The listing builds one solid part. Answer for the finished solid, in the listing's coordinates (mm). Coordinates: 2 decimals unless noted, no trailing zeros. Order: outer loops, then holes, each group sorted by start corner. A loop starts at its lowest first (then second) coordinate and runs counter-clockwise, first axis right, second up. Notation, with made-up numbers: (15.25, -28.5) -> (61.25, -28.5) arc R15 cw to (61.25, -11.5) -> close; hole circle Ø9 at (-29.75, 42.25). An arc over 180 degrees is marked (long way). One line per question, with ' | ' between items.
from build123d import *

# Parameters (mm, degrees)
SKETCH1_R           = 2.5
BOSS_EXTRUDE1_DEPTH = 4
CHAMFER1_SIZE       = 0.2


with BuildPart() as part:
    # Sketch1 → Boss-Extrude1 (new body)
    with BuildSketch(Plane(origin=(0, 0, 0), x_dir=(1, 0, 0), z_dir=(0, 1, 0))):
        Polygon((-2.309401077, 4), (-4.618802154, 0), (-2.309401077, -4), (2.309401077, -4), (4.618802154, 0), (2.309401077, 4), align=None)
        with Locations(Location((0, 0, 0), (0, 0, 270))):
            Circle(SKETCH1_R, mode=Mode.SUBTRACT)
    extrude(amount=BOSS_EXTRUDE1_DEPTH)

    # Chamfer1
    chamfer1_edges = [part.edges().sort_by_distance(p)[0] for p in [
        (0, 0, -2.5),
        (0, 4, -2.5),
    ]]
    chamfer(chamfer1_edges, length=CHAMFER1_SIZE)

    # Sketch2 → Cut-Revolve1 (revolve, cut)
    with BuildSketch(Plane.XY):
        Polygon((-4, 4), (-5, 3), (-5, 4), align=None)
        Polygon((-5, 0), (-4, 0), (-5, 1), align=None)
    revolve(axis=Axis((0, 0, 0), (0, 1, 0)), mode=Mode.SUBTRACT)


solid = part.part
Item 1: Section A-A, the plane y = 2.25 is taken. Give the vertices of the cut face in (x, z).
Computed values:
outline: (-4.62, 0) -> (-2.31, -4) -> (2.31, -4) -> (4.62, 0) -> (2.31, 4) -> (-2.31, 4) -> close; hole circle Ø5 at (0, 0)
Item 2: Find the intervals of material crossed by L1, parallel to Z at x = -1, y = 2.75; L2, parallel to X at y = 3, z = -1.75; L3, parallel to Z at x = -1.25, y = 3.1, in increasing order.
Computed values:
L1: z = -4 to -2.29, 2.29 to 4 | L2: x = -3.61 to -1.79, 1.79 to 3.61 | L3: z = -4 to -2.17, 2.17 to 4
Item 3: Determine the mould class of faces 1 (the face through (-2.44, 1.97, -0.54)), 2 (the face through (2.08, 0.15, -3.59)), 3 (the face through (4.2, 0.2, 0)) for opening direction Z: pulls with the +Z half, pulls with the -Z half, needs draft (parallel to the pull), parting line crosses it, or undercut.
Computed values:
face 1: undercut | face 2: pulls with the -Z half | face 3: parting line crosses it
